```python
from build123d import *

# Parameters (mm, degrees)
F0_R     = 30.3969812701
F1_DEPTH = 25.4
F3_DEPTH = 25.4
F4_R     = 7.532023706
F5_DEPTH = 25.4


# Not quite as in the source:
# - a feature names something its author has since deleted; it is built from what else it names


with BuildPart() as f1:
    # F0 (on Top) → F1 (new body)
    with BuildSketch(Plane.XY):
        Circle(F0_R)
    extrude(amount=F1_DEPTH)

    # F2 (on face) → F3 (cut)
    with BuildSketch(Plane.XY.offset(25.4)):
        Polygon((0, 0), (-30.3969812701, 0), (-30.3969812701, -28.1696463504), (-11.4213613388, -28.1696463504), align=None)
    extrude(amount=-F3_DEPTH, mode=Mode.SUBTRACT)

    # F4 (on face) → F5 (cut)
    with BuildSketch(Plane.XY.offset(25.4)):
        with Locations((-12.2123174369, 12.5044481829)):
            Circle(F4_R)
    extrude(amount=-F5_DEPTH, mode=Mode.SUBTRACT)


solid = f1.part
```
Could you check a few things on this model? Use its own coordinates, in mm. A direction names the side the tool comes from. Coordinates: 2 decimals unless noted, no trailing zeros. Write each loop counter-clockwise with the first axis right and the second up, starting at its lowest first coordinate (ties: lowest second). Pieces come first, ordered by that corner, then holes. Notation, with made-up numbers: (64, -39) -> (86, -39) arc R20 ccw to (86, -27) -> close; hole circle Ø2 at (12, -1.75). An arc over 180 degrees is marked (long way). One line per question, with ' | ' between items. Start each with the question number.
1. If we section it at B-B (z = 5.5): Please give me the cut outline in (x, y).
2. If we section it at D-D (x = 23): Please give me the cut outline in (y, z), and give its area (3 significant figures).
3. For faces 1 (the face through (-17.764, 17.595, 12.878)), 2 (the face through (-5.8, -14.3, 12.9)), which set-ups out of +Z, -Z, +X, -X, +Y, -Y let a thin tool reach every point of the face, with its end or its side?
4. Will these pins go through, and if not, where does the flat tip stop? P1, Ø3, axis at x = 1.5, z = 14, coming from the -Y side; P2, Ø4, axis at x = 4.5, z = 21.5, coming from the -Y side; P3, Ø4, axis at x = -17.5, z = 4.5, coming from the -Y side; P4, Ø2, axis at y = 15.5, z = 17, coming from the -X side.
5. Thinking about a two-plate mould opening in Y: for faces 3 (the face through (25.8, 16.07, 12.52)), 4 (the face through (6, 0, 0)), 5 (the face through (-15, 0, 13)), which applies, pulls with the +Y half, pulls with the -Y half, needs draft (parallel to the pull), parting line crosses it, or undercut?
6. Please list where these lines run through material, in increasing order: line 1 along Y through (x, z) = (-6.5, 4.5); line 2 along X through (y, z) = (13.5, 15.5); line 3 along X through (y, z) = (19, 20.75).
7. If we section it at A-A (y = 17): Please give me the cut outline in (x, z), and give its area (3 significant figures).
8. If we section it at C-C (y = -16): Please give me the cut outline in (x, z).
Return value:
1) outline: (-30.4, 0) -> (0, 0) -> (-11.42, -28.17) arc R30.4 ccw (long way) to start; hole circle Ø15.06 at (-12.21, 12.5)
2) outline: (-19.87, 0) -> (19.87, 0) -> (19.87, 25.4) -> (-19.87, 25.4) -> close | area: 1,010 mm²
3) face 1: +Z, -Z | face 2: +Z, -Z, -X
4) P1: stops at y = -30.4 | P2: stops at y = -30.29 | P3: stops at y = 0 | P4: stops at x = -26.72
5) face 3: parting line crosses it | face 4: needs draft | face 5: undercut
6) line 1: y = -29.69 to -16.03, 0 to 7.6, 17.41 to 29.69 | line 2: x = -27.23 to -19.68, -4.75 to 27.23 | line 3: x = -23.73 to -16.03, -8.4 to 23.73
7) outline: (-25.2, 0) -> (-18.26, 0) -> (-18.26, 25.4) -> (-25.2, 25.4) -> close; (-6.17, 0) -> (25.2, 0) -> (25.2, 25.4) -> (-6.17, 25.4) -> close | area: 973 mm²
8) outline: (-6.49, 0) -> (25.85, 0) -> (25.85, 25.4) -> (-6.49, 25.4) -> close
